Read the model definition and answer for the solid it produces. Units are mm, in the model's axes. A direction names the side the tool comes from. Coordinates: 2 decimals unless noted, no trailing zeros. Write each loop counter-clockwise with the first axis right and the second up, starting at its lowest first coordinate (ties: lowest second). Pieces come first, ordered by that corner, then holes. Notation, with made-up numbers: (-11.75, -15.75) - (12.25, -15.75) arc R18 ccw to (12.25, -10.75) - close; hole circle Ø4 at (-25.75, 15.5). An arc over 180 degrees is marked (long way). Use a Markdown table: item, result.
from build123d import *

# Parameters (mm, degrees)
SKETCH_2_W               = 1.5
SKETCH_2_H               = 1.2
CUT_EXTRUDE_1_DEPTH      = 4
CUT_EXTRUDE_1_DEPTH_BACK = 4
CHAMFER_1_SIZE           = 0.4
FILLET_1_R               = 1
FILLET_2_R               = 0.4


with BuildPart() as part:
    # Эскиз1 → Повернуть1 (revolve)
    with BuildSketch(Plane(origin=(0, 0, 0), x_dir=(1, 0, 0), z_dir=(0, 1, 0))):
        Polygon((0, 0), (-3, 0), (-3, 1.8), (-1.5, 1.8), (-1.5, 21.8), (0, 21.8), align=None)
    revolve(axis=Axis((0, 0, -21.8), (0, 0, 1)))

    # Эскиз2 → Вырез-Вытянуть1 (cut, two sides)
    with BuildSketch(Plane(origin=(0, 0, 0), x_dir=(0, 0, -1), z_dir=(1, 0, 0))) as cut_extrude_1_sk:
        with Locations((0.75, 0)):
            Rectangle(SKETCH_2_W, SKETCH_2_H)
    extrude(amount=CUT_EXTRUDE_1_DEPTH, mode=Mode.SUBTRACT)
    extrude(cut_extrude_1_sk.sketch, amount=-CUT_EXTRUDE_1_DEPTH_BACK, mode=Mode.SUBTRACT)

    # Фаска1
    chamfer_1_edges = [part.edges().sort_by_distance(p)[0] for p in [
        (1.5, 0, -21.8),
    ]]
    chamfer(chamfer_1_edges, length=CHAMFER_1_SIZE)

    # Скругление1
    fillet_1_edges = [part.edges().sort_by_distance(p)[0] for p in [
        (0, 3, 0),
        (0, -3, 0),
    ]]
    fillet(fillet_1_edges, radius=FILLET_1_R)

    # Скругление2
    fillet_2_edges = [part.edges().sort_by_distance(p)[0] for p in [
        (1.5, 0, -1.8),
    ]]
    fillet(fillet_2_edges, radius=FILLET_2_R)


solid = part.part
(1) For faces 1 (the flat face through (-1, 2, -1.8)), 2 (the cylindrical face through (-2.77, 1.15, -1.41)), 3 (the flat face through (0, 0.6, -1)), determine the directions among +Z, -Z, +X, -X, +Y, -Y from which every point of the face is accessible in a straight line to the end or side of a thin tool.
Report:
| item | result |
|---|---|
| face 1 | -Z |
| face 2 | +Z, -Z |
| face 3 | +Z, +X, -X |
(2) The mould has two halves that part along Y. Classify faces 4 (the cylindrical face through (1.5, -0.07, -11.93)), 5 (the flat face through (0, 1, 0)), 6 (the flat face through (0, -0.6, -1)): pulls with the +Y half, pulls with the -Y half, needs draft (parallel to the pull), parting line crosses it, or undercut.
Report:
| item | result |
|---|---|
| face 4 | parting line crosses it |
| face 5 | needs draft |
| face 6 | undercut |
(3) A cutting plane is placed at B-B, the plane x = 0. Write down the section's boundary in (y, z), and give its area (3 significant figures).
Report:
| item | result |
|---|---|
| outline | (-3, -1.8) - (-1.9, -1.8) arc R0.4 cw to (-1.5, -2.2) - (-1.5, -21.4) - (-1.1, -21.8) - (1.1, -21.8) - (1.5, -21.4) - (1.5, -2.2) arc R0.4 cw to (1.9, -1.8) - (3, -1.8) - (3, -1) arc R1 ccw to (2, 0) - (0.6, 0) - (0.6, -1.5) - (-0.6, -1.5) - (-0.6, 0) - (-2, 0) arc R1 ccw to (-3, -1) - close |
| area | 68.5 mm² |
(4) Straight lines are drawn through the part: L1, parallel to Z at x = 1.6, y = -1.25; L2, parallel to Z at x = 2.6, y = 0; L3, parallel to X at y = -1, z = -13.5. For each, find the intervals that lie inside material, in ascending order.
Report:
| item | result |
|---|---|
| L1 | z = -1.8 to 0 |
| L2 | z = -1.8 to -1.5 |
| L3 | x = -1.12 to 1.12 |
(5) A cutting plane is placed at A-A, the plane y = 0. Write down the section's boundary in (x, z), and give its area (3 significant figures).
Report:
| item | result |
|---|---|
| outline | (-3, -1.8) - (-1.9, -1.8) arc R0.4 cw to (-1.5, -2.2) - (-1.5, -21.4) - (-1.1, -21.8) - (1.1, -21.8) - (1.5, -21.4) - (1.5, -2.2) arc R0.4 cw to (1.9, -1.8) - (3, -1.8) - (3, -1.5) - (-3, -1.5) - close |
| area | 61.7 mm² |
(6) Each of these flat-tipped pins is pushed along its axis until it touches: P1, Ø1, axis at x = 0, z = -18, coming from the +Y side; P2, Ø3, axis at y = 1.5, z = -10.5, coming from the -X side; P3, Ø2, axis at x = 0, z = -17, coming from the -Y side; P4, Ø0.8, axis at x = -0.5, z = -1, coming from the +Y side. Where does it stop, or does it pass through?
Report:
| item | result |
|---|---|
| P1 | stops at y = 1.5 |
| P2 | stops at x = -1.5 |
| P3 | stops at y = -1.5 |
| P4 | stops at y = 3 |
(7) A cutting plane is placed at C-C, the plane z = -3.5. Write down the section's boundary in (x, y), and give its area (3 significant figures).
Report:
| item | result |
|---|---|
| outline | circle Ø3 at (0, 0) |
| area | 7.07 mm² |
